Job drawing, mm, ordinate dimensions from the low corner. One solid piece. Give positions to 0.01 mm unless a question says otherwise; leave off trailing zeros. Order: outer loops, then holes, each group sorted by start corner. A loop starts at its lowest first (then second) coordinate and runs counter-clockwise, first axis right, second up. Notation, with made-up numbers: M 7.25,48.5 L 47.25,48.5 A30 cw 47.25,72.5 Z; hole C 62.5,39 d11. An arc over 180 degrees is marked long. One line per question, with ' | ' between items.
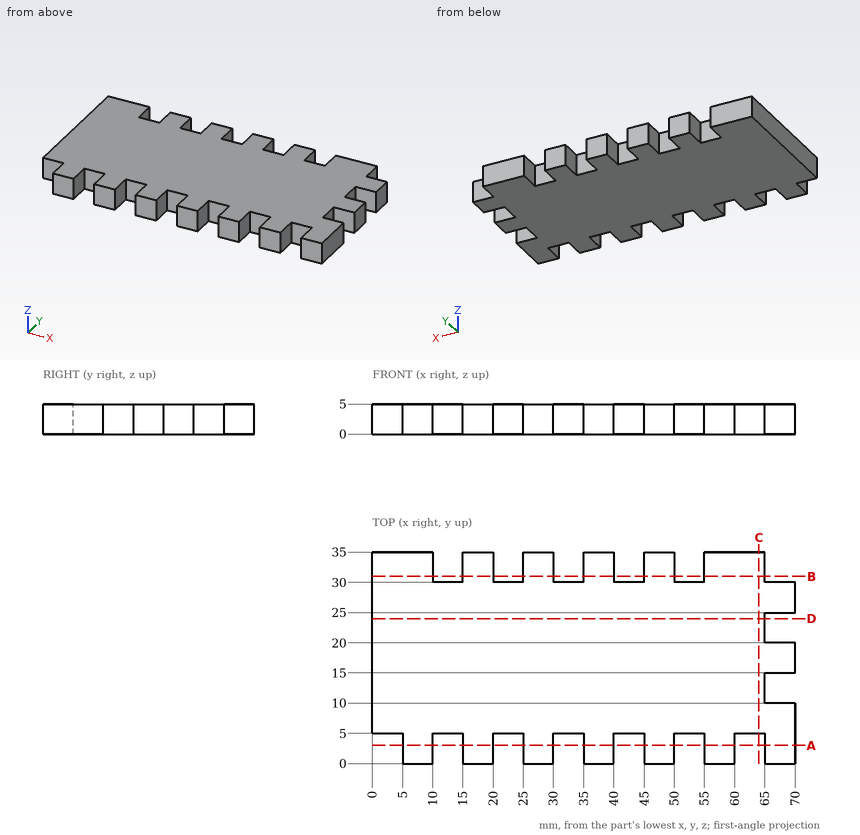
1. Slice it at B-B on y = 31. Give the cut face in (x, z), then the cut area to 3 significant figures.
Worked out:
outline: M 0,0 L 10,0 L 10,5 L 0,5 Z; M 15,0 L 20,0 L 20,5 L 15,5 Z; M 25,0 L 30,0 L 30,5 L 25,5 Z; M 35,0 L 40,0 L 40,5 L 35,5 Z; M 45,0 L 50,0 L 50,5 L 45,5 Z; M 55,0 L 65,0 L 65,5 L 55,5 Z | area: 200 mm2
2. Slice it at D-D on y = 24. Give the cut face in (x, z).
Worked out:
outline: M 0,0 L 65,0 L 65,5 L 0,5 Z
3. Slice it at C-C on x = 64. Give the cut face in (y, z), then the cut area to 3 significant figures.
Worked out:
outline: M 5,0 L 35,0 L 35,5 L 5,5 Z | area: 150 mm2
4. Slice it at A-A on y = 3. Give the cut face in (x, z).
Worked out:
outline: M 5,0 L 10,0 L 10,5 L 5,5 Z; M 15,0 L 20,0 L 20,5 L 15,5 Z; M 25,0 L 30,0 L 30,5 L 25,5 Z; M 35,0 L 40,0 L 40,5 L 35,5 Z; M 45,0 L 50,0 L 50,5 L 45,5 Z; M 55,0 L 60,0 L 60,5 L 55,5 Z; M 65,0 L 70,0 L 70,5 L 65,5 Z
5. Probe L1, parallel to Y at x = 67, z = 0.95; L2, parallel to X at y = 23, z = 2.05; L3, parallel to Y at x = 14, z = 1.6. List the from-to ranges inside material, lowest first. Write a range as from..to.
Worked out:
L1: y = 0..10, 15..20, 25..30 | L2: x = 0..65 | L3: y = 5..30
6. Drop flat-ended pins along their axis: pin 1 (2.5 mm diameter, centred on x = 67.5, z = 2, fed in from +Y); pin 2 (2.5 mm diameter, centred on y = 32, z = 2, fed in from +X); pin 3 (2.5 mm diameter, centred on y = 2.5, z = 3.5, fed in from -X). Give the stop position or say it passes through.
Worked out:
pin 1: stops at y = 30 | pin 2: stops at x = 65 | pin 3: stops at x = 5
